```python
from build123d import *

# Parameters (mm, degrees)
SKETCH_1_W          = 19
SKETCH_1_H          = 42
SKETCH_1_R          = 1.65
EXTRUDE_1_DEPTH     = 3
SKETCH_2_R          = 2.5
CUT_EXTRUDE_1_DEPTH = 4
FILLET_1_R          = 2
FILLET_2_R          = 2


with BuildPart() as part:
    # 草图1 → 凸台-拉伸1 (new body)
    with BuildSketch(Plane.XY):
        Rectangle(SKETCH_1_W, SKETCH_1_H)
        with Locations((-6.5, 18)):
            Circle(SKETCH_1_R, mode=Mode.SUBTRACT)
        with Locations((-6.5, 5.5)):
            Circle(SKETCH_1_R, mode=Mode.SUBTRACT)
        with Locations((4.5, -10)):
            Circle(SKETCH_1_R, mode=Mode.SUBTRACT)
        with Locations((4.5, -18)):
            Circle(SKETCH_1_R, mode=Mode.SUBTRACT)
        with Locations((4.5, 18)):
            Circle(SKETCH_1_R, mode=Mode.SUBTRACT)
        with Locations((4.5, 5.5)):
            Circle(SKETCH_1_R, mode=Mode.SUBTRACT)
    extrude(amount=EXTRUDE_1_DEPTH)

    # 草图2 → 切除-拉伸1 (cut, through all)
    with BuildSketch(Plane.XY.offset(3)):
        with Locations((-9.5, 11.5)):
            Circle(SKETCH_2_R)
    extrude(amount=-CUT_EXTRUDE_1_DEPTH, mode=Mode.SUBTRACT)

    # 圆角1
    fillet_1_edges = [part.edges().sort_by_distance(p)[0] for p in [
        (-9.5, 9, 1.5),
        (-9.5, 14, 1.5),
    ]]
    fillet(fillet_1_edges, radius=FILLET_1_R)

    # 圆角2
    fillet_2_edges = [part.edges().sort_by_distance(p)[0] for p in [
        (9.5, -21, 1.5),
        (-9.5, -21, 1.5),
        (-9.5, 21, 1.5),
        (9.5, 21, 1.5),
    ]]
    fillet(fillet_2_edges, radius=FILLET_2_R)


solid = part.part
```
Model file for the job. Use its own axes, mm. A direction names the side the tool comes from. Coordinates: 2 decimals unless noted, no trailing zeros. Write each loop counter-clockwise with the first axis right and the second up, starting at its lowest first coordinate (ties: lowest second). Pieces come first, ordered by that corner, then holes. Notation, with made-up numbers: (43.25, -1) - (79.25, -1) arc R12 ccw to (79.25, 4) - close; hole circle Ø7 at (-32, 0). An arc over 180 degrees is marked (long way). One line per item, written item: value. Start each with the question number.
1. Tool access for faces 1 (the cylindrical face through (-9.208, 8.51, 1.521)), 2 (the cylindrical face through (3.19, -11, 1.48)): list every direction of +Z, -Z, +X, -X, +Y, -Y with a clear straight run to the whole face (end or side of a thin tool).
2. Slice it at C-C (x = -6.5). Write the cut outline in (y, z), plus the area to 3 significant figures.
3. Mould opens along X. For faces 3 (the cylindrical face through (-7.81, 4.5, 1.48)), 4 (the cylindrical face through (-9.208, 14.49, 1.521)), 5 (the flat face through (0, 0, 0)) say: released by +X, released by -X, zero draft, split by the parting line, or undercut.
4. Slice it at B-B (z = 2). Write the cut outline in (x, y).
5. Probe line 1 (Y direction, x = 4.5, z = 0.95); line 2 (Y direction, x = -6.5, z = 1.1); line 3 (Y direction, x = 6, z = 0.25). List the from-to ranges inside material, lowest first. Write a range as from..to.
6. Slice it at D-D (x = 4.5). Write the cut outline in (y, z), plus the area to 3 significant figures.
7. Slice it at A-A (y = -18). Write the cut outline in (x, z), plus the area to 3 significant figures.
8. Flat gauge pin, fed straight in: pin 1 (5.5 mm diameter, centred on x = 4.5, y = -18, fed in from -Z). Where does the tip first touch, or does it go through?
Answers below:
1. face 1: +Z, -Z, -X
1. face 2: +Z, -Z
2. outline: (-21, 0) - (3.85, 0) - (3.85, 3) - (-21, 3) - close; (7.15, 0) - (16.35, 0) - (16.35, 3) - (7.15, 3) - close; (19.65, 0) - (21, 0) - (21, 3) - (19.65, 3) - close
2. area: 106 mm^2
3. face 3: undercut
3. face 4: released by -X
3. face 5: zero draft
4. outline: (-9.5, -19) arc R2 ccw to (-7.5, -21) - (7.5, -21) arc R2 ccw to (9.5, -19) - (9.5, 19) arc R2 ccw to (7.5, 21) - (-7.5, 21) arc R2 ccw to (-9.5, 19) - (-9.5, 15.53) arc R2 ccw to (-8.39, 13.74) arc R2.5 cw to (-8.39, 9.26) arc R2 ccw to (-9.5, 7.47) - close; hole circle Ø3.3 at (-6.5, 5.5); hole circle Ø3.3 at (-6.5, 18); hole circle Ø3.3 at (4.5, -18); hole circle Ø3.3 at (4.5, -10); hole circle Ø3.3 at (4.5, 5.5); hole circle Ø3.3 at (4.5, 18)
5. line 1: y = -21..-19.65, -16.35..-11.65, -8.35..3.85, 7.15..16.35, 19.65..21
5. line 2: y = -21..3.85, 7.15..16.35, 19.65..21
5. line 3: y = -21..-18.69, -17.31..-10.69, -9.31..4.81, 6.19..17.31, 18.69..21
6. outline: (-21, 0) - (-19.65, 0) - (-19.65, 3) - (-21, 3) - close; (-16.35, 0) - (-11.65, 0) - (-11.65, 3) - (-16.35, 3) - close; (-8.35, 0) - (3.85, 0) - (3.85, 3) - (-8.35, 3) - close; (7.15, 0) - (16.35, 0) - (16.35, 3) - (7.15, 3) - close; (19.65, 0) - (21, 0) - (21, 3) - (19.65, 3) - close
6. area: 86.4 mm^2
7. outline: (-9.5, 0) - (2.85, 0) - (2.85, 3) - (-9.5, 3) - close; (6.15, 0) - (9.5, 0) - (9.5, 3) - (6.15, 3) - close
7. area: 47.1 mm^2
8. pin 1: stops at z = 0
